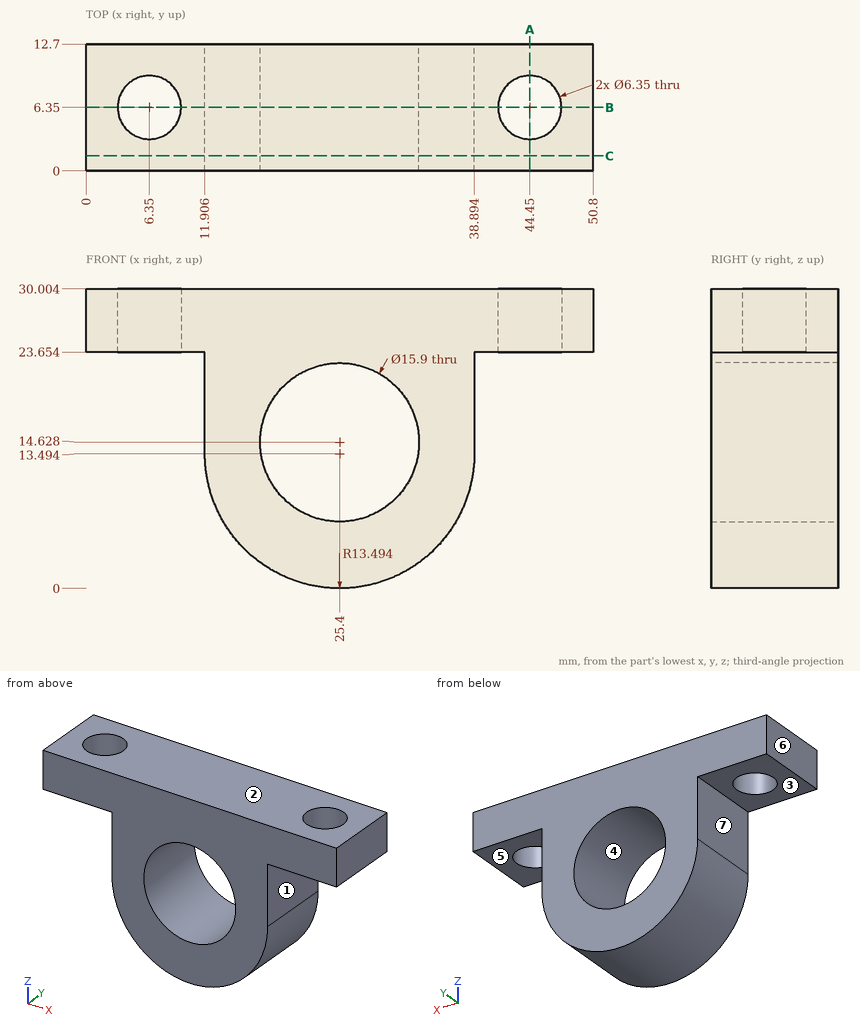
The figure shows three views and two pictorial views of one solid part (mm, origin at its lowest corner). Answer the questions. A direction names the side the tool comes from. Coordinates: 2 decimals unless noted, no trailing zeros. Loops run counter-clockwise (first coordinate to the right, second up) from the corner with the lowest first, then second, coordinate; pieces in that order, holes last. Notation, with made-up numbers: (8, 38.5) - (36, 38.5) arc R11 ccw to (36, 46.5) - close; hole circle Ø8 at (77, 35). An arc over 180 degrees is marked (long way). Use a Markdown table: item, result. Add a question column.
1) Find the intervals of material crossed by line 1 (Y direction, x = 44.45, z = 26.25) (1 decimal); line 2 (X direction, y = 3.5, z = 28.5); line 3 (X direction, y = 5.75, z = 25.5), in increasing order.
2) For the marked faces 5, 6 and 7, determine the directions among +Z, -Z, +X, -X, +Y, -Y from which every point of the face is accessible in a straight line to the end or side of a thin tool.
3) Given pin 1 (7.5 mm diameter, centred on x = 6.35, y = 6.35, fed in from -Z); pin 2 (1.5 mm diameter, centred on y = 10.5, z = 20.5, fed in from -X); pin 3 (5 mm diameter, centred on y = 4, z = 20.5, fed in from +X), each flat-ended and moving along its own axis, determine where each tip first touches the part or whether it passes through.
4) The part is cut by section A-A, the plane x = 44.45. Give the vertices of the cut face in (y, z) (1 decimal).
5) The part is cut by section C-C, the plane y = 1.5. Give the vertices of the cut face in (x, z), and give its area (3 significant figures).
6) The part is cut by section B-B, the plane y = 6.35. State how many separate pieces and enclosed holes the cut face has.
7) The mould has two halves that part along Z. Classify the marked faces 1, 2, 3 and 4: released by +Z, released by -Z, zero draft, split by the parting line, or undercut.
Here are the results:
| question | item | result |
|---|---|---|
| 1 | line 1 | y = 0 to 3.2, 9.5 to 12.7 |
| 1 | line 2 | x = 0 to 4.95, 7.75 to 43.05, 45.85 to 50.8 |
| 1 | line 3 | x = 0 to 3.23, 9.47 to 41.33, 47.57 to 50.8 |
| 2 | face 5 | -Z, +X, +Y, -Y |
| 2 | face 6 | +Z, -Z, -X, +Y, -Y |
| 2 | face 7 | -Z, -X, +Y, -Y |
| 3 | pin 1 | stops at z = 23.65 |
| 3 | pin 2 | stops at x = 11.91 |
| 3 | pin 3 | stops at x = 38.89 |
| 4 | outline | (0, 23.7) - (3.2, 23.7) - (3.2, 30) - (0, 30) - close; (9.5, 23.7) - (12.7, 23.7) - (12.7, 30) - (9.5, 30) - close |
| 5 | outline | (0, 23.65) - (11.91, 23.65) - (11.91, 13.49) arc R13.49 ccw to (38.89, 13.49) - (38.89, 23.65) - (50.8, 23.65) - (50.8, 30) - (0, 30) - close; hole circle Ø15.9 at (25.4, 14.63) |
| 5 | area | 684 mm^2 |
| 6 | separate pieces | 3 |
| 6 | enclosed holes | 1 |
| 7 | face 1 | zero draft |
| 7 | face 2 | released by +Z |
| 7 | face 3 | released by -Z |
| 7 | face 4 | undercut |
